```python
from build123d import *

# Parameters (mm, degrees)
SKETCH1_W           = 27
SKETCH1_H           = 37
SKETCH1_R           = 8.05
SKETCH1_R_2         = 1.5
SKETCH1_R_3         = 1.75
BOSS_EXTRUDE1_DEPTH = 5
SKETCH1_4_R         = 1.5
BOSS_EXTRUDE3_DEPTH = 4.95
SKETCH1_5_R         = 8.05
SKETCH1_5_R_2       = 2.8
BOSS_EXTRUDE4_DEPTH = 2
FILLET1_R           = 10
BOSS_EXTRUDE5_START = 17
BOSS_EXTRUDE5_DEPTH = 17


with BuildPart() as part:
    # Sketch1 → Boss-Extrude1 (new body)
    with BuildSketch(Plane(origin=(0, 0, 0), x_dir=(1, 0, 0), z_dir=(0, 1, 0))):
        with Locations((0, 5)):
            Rectangle(SKETCH1_W, SKETCH1_H)
        with Locations(Location((0, 0, 0), (0, 0, 270))):
            Circle(SKETCH1_R, mode=Mode.SUBTRACT)
        with Locations(Location((0, 13.337, 0), (0, 0, 270))):
            Circle(SKETCH1_R_2, mode=Mode.SUBTRACT)
        with Locations(Location((-9.5, 8, 0), (0, 0, 270))):
            Circle(SKETCH1_R_3, mode=Mode.SUBTRACT)
        with Locations(Location((9.5, 8, 0), (0, 0, 270))):
            Circle(SKETCH1_R_3, mode=Mode.SUBTRACT)
    extrude(amount=BOSS_EXTRUDE1_DEPTH)

    # Sketch1<4> → Boss-Extrude3 (add)
    with BuildSketch(Plane(origin=(0, 0, 0), x_dir=(1, 0, 0), z_dir=(0, 1, 0))):
        with Locations(Location((0, 13.337, 0), (0, 0, 270))):
            Circle(SKETCH1_4_R)
    extrude(amount=BOSS_EXTRUDE3_DEPTH)

    # Sketch1<5> → Boss-Extrude4 (add)
    # profile 1 of 3: a face of its own
    with BuildSketch(Plane(origin=(0, 0, 0), x_dir=(1, 0, 0), z_dir=(0, 1, 0))):
        with Locations(Location((0, 0, 0), (0, 0, 270))):
            Circle(SKETCH1_5_R)
        with Locations(Location((0, 0, 0), (0, 0, 270))):
            Circle(SKETCH1_5_R_2, mode=Mode.SUBTRACT)
    # profile 2 of 3: a face of its own
    with BuildSketch(Plane(origin=(0, 0, 0), x_dir=(1, 0, 0), z_dir=(0, 1, 0))):
        with BuildLine():
            ThreePointArc((-5.45, 5.924525297), (-5.753510872, 5.630240905), (-6.041153839, 5.320428582))
            Line((-6.041153839, 5.320428582), (-5.45, 5.66173141))
            Line((-5.45, 5.66173141), (-5.45, 5.924525297))
        make_face()
    # profile 3 of 3: a face of its own
    with BuildSketch(Plane(origin=(0, 0, 0), x_dir=(1, 0, 0), z_dir=(0, 1, 0))):
        with BuildLine():
            Line((5.45, 5.66173141), (6.041153839, 5.320428582))
            ThreePointArc((6.041153839, 5.320428582), (5.753510872, 5.630240905), (5.45, 5.924525297))
            Line((5.45, 5.924525297), (5.45, 5.66173141))
        make_face()
    extrude(amount=BOSS_EXTRUDE4_DEPTH)

    # Fillet1
    fillet1_edges = [part.edges().sort_by_distance(p)[0] for p in [
        (-13.5, 2.5, -23.5),
        (13.5, 2.5, -23.5),
        (13.5, 2.5, 13.5),
        (-13.5, 2.5, 13.5),
    ]]
    fillet(fillet1_edges, radius=FILLET1_R)

    # Sketch2 → Boss-Extrude5 (add)
    with BuildSketch(Plane(origin=(0, 5, 0), x_dir=(1, 0, 0), z_dir=(0, 1, 0)).offset(BOSS_EXTRUDE5_START)):
        with BuildLine():
            Line((13.5, -3.5), (13.5, 13.5))
            ThreePointArc((13.5, 13.5), (10.571067812, 20.571067812), (3.5, 23.5))
            Line((3.5, 23.5), (-3.5, 23.5))
            ThreePointArc((-3.5, 23.5), (-10.571067812, 20.571067812), (-13.5, 13.5))
            Line((-13.5, 13.5), (-13.5, -3.5))
            ThreePointArc((-13.5, -3.5), (-10.571067812, -10.571067812), (-3.5, -13.5))
            Line((-3.5, -13.5), (3.5, -13.5))
            ThreePointArc((3.5, -13.5), (10.571067812, -10.571067812), (13.5, -3.5))
        make_face()
        with BuildLine():
            Line((-12.3, 13.5), (-12.3, -3.5))
            ThreePointArc((-12.3, -3.5), (-9.722539674, -9.722539674), (-3.5, -12.3))
            Line((-3.5, -12.3), (3.5, -12.3))
            ThreePointArc((3.5, -12.3), (9.722539674, -9.722539674), (12.3, -3.5))
            Line((12.3, -3.5), (12.3, 13.5))
            ThreePointArc((12.3, 13.5), (9.722539674, 19.722539674), (3.5, 22.3))
            Line((3.5, 22.3), (-3.5, 22.3))
            ThreePointArc((-3.5, 22.3), (-9.722539674, 19.722539674), (-12.3, 13.5))
        make_face(mode=Mode.SUBTRACT)
    extrude(amount=-BOSS_EXTRUDE5_DEPTH)


solid = part.part
```
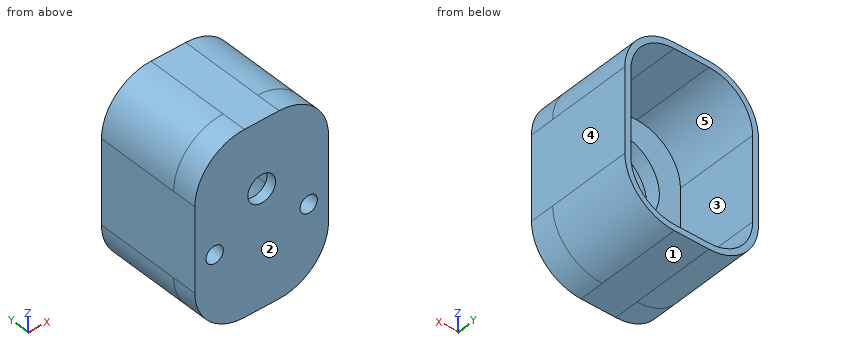
Geometry: final body of the model. Coordinates: model frame, mm. Face numbers are marked on the shaded views. A direction names the side the tool comes from. Round coordinates to 2 decimals unless told otherwise and drop trailing zeros. Write each loop counter-clockwise with the first axis right and the second up, starting at its lowest first coordinate (ties: lowest second). Pieces come first, ordered by that corner, then holes.
Item 1: Section query C-C (z = 0). Return loops of the section in (x, y).
Item 2: Material intervals for L1, parallel to X at y = 20.25, z = 0.5; L2, parallel to X at y = 1.2, z = 0; L3, parallel to Z at x = -0.75, y = 5.25, sorted ascending.
Item 3: Set-up query: the marked faces 4 and 5. Return all of +Z, -Z, +X, -X, +Y, -Y with unobstructed straight access to the full face (end or side cutting, diameter ignored); none if empty.
Item 4: Pin query (flat end, axial travel): P1, Ø10, axis at x = -10.5, y = 16, coming from the -Z side; P2, Ø1.5, axis at x = 0.5, z = -14, coming from the +Y side; P3, Ø10, axis at x = -2.5, z = 1, coming from the +Y side. Return the tip coordinate at first contact, or that it passes through.
Item 5: Section query B-B (y = 16.5). Return loops of the section in (x, z).
Item 6: Mould query, pull axis Z, two halves, no side actions, for the marked faces 1, 2 and 3. Classes: +Z half, -Z half, draft (parallel to the pull), parting line (faces both ways), or undercut.
Item 7: Section query D-D (y = 3). Return loops of the section in (x, z), plus the area to 3 significant figures.
Item 8: Section query A-A (x = 0). Return loops of the section in (y, z), plus the area to 3 significant figures.
Completed:
1. outline: (-13.5, 0) - (-2.8, 0) - (-2.8, 2) - (-8.05, 2) - (-8.05, 5) - (-12.3, 5) - (-12.3, 22) - (-13.5, 22) - close; (2.8, 0) - (13.5, 0) - (13.5, 22) - (12.3, 22) - (12.3, 5) - (8.05, 5) - (8.05, 2) - (2.8, 2) - close
2. L1: x = -13.5 to -12.3, 12.3 to 13.5
2. L2: x = -13.5 to -2.8, 2.8 to 13.5
2. L3: z = -23.5 to -22.3, 12.3 to 13.5
3. face 4: +Z, -Z, +X, +Y, -Y
3. face 5: +Y
4. P1: stops at z = -23.3
4. P2: stops at y = 5
4. P3: stops at y = 2
5. outline: (-13.5, -13.5) arc R10 ccw to (-3.5, -23.5) - (3.5, -23.5) arc R10 ccw to (13.5, -13.5) - (13.5, 3.5) arc R10 ccw to (3.5, 13.5) - (-3.5, 13.5) arc R10 ccw to (-13.5, 3.5) - close; hole (-12.3, -13.5) arc R8.8 ccw to (-3.5, -22.3) - (3.5, -22.3) arc R8.8 ccw to (12.3, -13.5) - (12.3, 3.5) arc R8.8 ccw to (3.5, 12.3) - (-3.5, 12.3) arc R8.8 ccw to (-12.3, 3.5) - close
6. face 1: -Z half
6. face 2: draft
6. face 3: undercut
7. outline: (-13.5, -13.5) arc R10 ccw to (-3.5, -23.5) - (3.5, -23.5) arc R10 ccw to (13.5, -13.5) - (13.5, 3.5) arc R10 ccw to (3.5, 13.5) - (-3.5, 13.5) arc R10 ccw to (-13.5, 3.5) - close; hole circle Ø3.5 at (-9.5, -8); hole circle Ø16.1 at (0, 0); hole circle Ø3.5 at (9.5, -8)
7. area: 690 mm2
8. outline: (0, -23.5) - (22, -23.5) - (22, -22.3) - (5, -22.3) - (5, -14.84) - (4.95, -14.84) - (4.95, -11.84) - (5, -11.84) - (5, -8.05) - (2, -8.05) - (2, -2.8) - (0, -2.8) - close; (0, 2.8) - (2, 2.8) - (2, 8.05) - (5, 8.05) - (5, 12.3) - (22, 12.3) - (22, 13.5) - (0, 13.5) - close
8. area: 166 mm2
